Can you work these out from the model? Positions are in its coordinate system, mm. A direction names the side the tool comes from. Give positions to 0.01 mm unless a question says otherwise; leave off trailing zeros. Loops run counter-clockwise (first coordinate to the right, second up) from the corner with the lowest first, then second, coordinate; pieces in that order, holes last.
Autodesk Inventor part; units mm, degrees
ref_plane "YZ Plane" through (0, 0, 0) normal (1, 0, 0) x (0, 1, 0)
ref_plane "XZ Plane" through (0, 0, 0) normal (0, 1, 0) x (-1, 0, 0)
ref_plane "XY Plane" through (0, 0, 0) normal (0, 0, 1) x (1, 0, 0)
sketch "Sketch1" plane through (0, 0, 0) normal (0, 0, 1) x (1, 0, 0)
  circle A0 centre (0, 0) radius 2.54
  circle A1 centre (0, 0) radius 15.875
  dimension "d0" = 5.08
  dimension "d1" = 31.75
extrude "Extrusion1" add sketch "Sketch1" along normal blind 6.35
sketch "Sketch2" plane through (0, 0, 6.35) normal (0, 0, 1) x (1, 0, 0)
  circle A0 centre (0, 0) radius 11
  circle A1 centre (0, 0) radius 3.9625
  circle A2 centre (0, -8) radius 1.6025
  circle A3 centre (8, 0) radius 1.6025
  circle A4 centre (-8, 0) radius 1.6025
  circle A5 centre (0, 8) radius 1.6025
extrude "Extrusion2" cut sketch "Sketch2" against normal blind 6.35 contours A2 | A3 | A4 | A5
sketch "Sketch4" plane through (0, 0, 6.35) normal (0, 0, 1) x (1, 0, 0)
  circle A0 centre (0, 0) radius 2.54
  circle A1 centre (0, 0) radius 15.875
  circle A2 centre (0, 0) radius 3.9624
  dimension "d6" = 7.9248
extrude "Extrusion3" cut sketch "Sketch4" against normal blind 3.175 contours A2
properties part number "end piece for spool"
(1) Which directions (+Z, -Z, +X, -X, +Y, -Y) give clear straight access to the entire face, cutting with the end or side of a thin tool? Please do faces 5 (the cylindrical face through (1.48, -8.61, 3.22)), 6 (the cylindrical face through (-0.52, 3.93, 4.78)).
Returned:
face 5: +Z, -Z
face 6: +Z
(2) Suppose I cut it at D-D on x = -7. List the corners of the cut face in (y, z) for me, plus the area to 3 significant figures.
Returned:
outline: (-14.25, 0) - (-1.25, 0) - (-1.25, 6.35) - (-14.25, 6.35) - close; (1.25, 0) - (14.25, 0) - (14.25, 6.35) - (1.25, 6.35) - close
area: 165 mm2
(3) Will these pins go through, and if not, where does the flat tip stop? P1, Ø4, axis at x = -1, y = 0, coming from the +Z side (3 decimals); P2, Ø2.5, axis at x = 8, y = 0, coming from the -Z side.
Returned:
P1: stops at z = 3.175
P2: passes through
(4) Suppose I cut it at A-A on x = 0. Give the number of separate pieces and of enclosed holes in the cut face, plus the area to 3 significant figures.
Returned:
separate pieces: 4
enclosed holes: 0
area: 120 mm2
(5) Thinking about a two-plate mould opening in X: for faces 1 (the cylindrical face through (-0.33, -2.52, 1.57)), 2 (the flat face through (3, -3, 6.35)), 3 (the cylindrical face through (-0.21, 9.59, 3.22)), 4 (the cylindrical face through (-3.441, 15.497, 3.131)), which applies, pulls with the +X half, pulls with the -X half, needs draft (parallel to the pull), parting line crosses it, or undercut?
Returned:
face 1: undercut
face 2: needs draft
face 3: undercut
face 4: parting line crosses it
(6) Please list where these lines run through material, in increasing order: probe 1 along Y at (x, z) = (0, 1.9) (1 decimal); probe 2 along Y at (x, z) = (0, 4.75) (1 decimal); probe 3 along X at (y, z) = (-1, 5.5).
Returned:
probe 1: y = -15.9 to -9.6, -6.4 to -2.5, 2.5 to 6.4, 9.6 to 15.9
probe 2: y = -15.9 to -9.6, -6.4 to -4, 4 to 6.4, 9.6 to 15.9
probe 3: x = -15.84 to -9.25, -6.75 to -3.83, 3.83 to 6.75, 9.25 to 15.84
